Check sheet for the modelled part. Datum: model origin and axes. Units: mm. Give positions to 0.01 mm unless a question says otherwise; leave off trailing zeros. Order: outer loops, then holes, each group sorted by start corner. A loop starts at its lowest first (then second) coordinate and runs counter-clockwise, first axis right, second up.
from build123d import *

# Parameters (mm, degrees)
BOSS_EXTRUDE1_DEPTH = 4
CUT_EXTRUDE1_DEPTH  = 5


with BuildPart() as part:
    # Sketch1 → Boss-Extrude1 (new body)
    with BuildSketch(Plane(origin=(0, 0, 0), x_dir=(1, 0, 0), z_dir=(0, 1, 0))):
        Polygon((-65.5, 20), (-70, 20), (-70, -19.415515436), (-65.5, -19.415515436), (-65.5, -60), (65.5, -60), (65.5, -19.415515436), (70, -19.415515436), (70, 20), (65.5, 20), (65.5, 60), (-65.5, 60), align=None)
    extrude(amount=BOSS_EXTRUDE1_DEPTH)

    # Sketch2 → Cut-Extrude1 (cut)
    with BuildSketch(Plane(origin=(0, 4, 0), x_dir=(1, 0, 0), z_dir=(0, 1, 0))):
        with BuildLine():
            Line((-53.5, -20), (12.5, -20))
            ThreePointArc((12.5, -20), (13.914213562, -19.414213562), (14.5, -18))
            Line((14.5, -18), (14.5, 48))
            ThreePointArc((14.5, 48), (13.914213562, 49.414213562), (12.5, 50))
            Line((12.5, 50), (-53.5, 50))
            ThreePointArc((-53.5, 50), (-54.914213562, 49.414213562), (-55.5, 48))
            Line((-55.5, 48), (-55.5, -18))
            ThreePointArc((-55.5, -18), (-54.914213562, -19.414213562), (-53.5, -20))
        make_face()
        with BuildLine():
            Line((22.5, -44), (38.5, -44))
            ThreePointArc((38.5, -44), (39.207106781, -43.707106781), (39.5, -43))
            Line((39.5, -43), (39.5, -37))
            ThreePointArc((39.5, -37), (39.207106781, -36.292893219), (38.5, -36))
            Line((38.5, -36), (22.5, -36))
            ThreePointArc((22.5, -36), (21.792893219, -36.292893219), (21.5, -37))
            Line((21.5, -37), (21.5, -43))
            ThreePointArc((21.5, -43), (21.792893219, -43.707106781), (22.5, -44))
        make_face()
    extrude(amount=-CUT_EXTRUDE1_DEPTH, mode=Mode.SUBTRACT)


solid = part.part
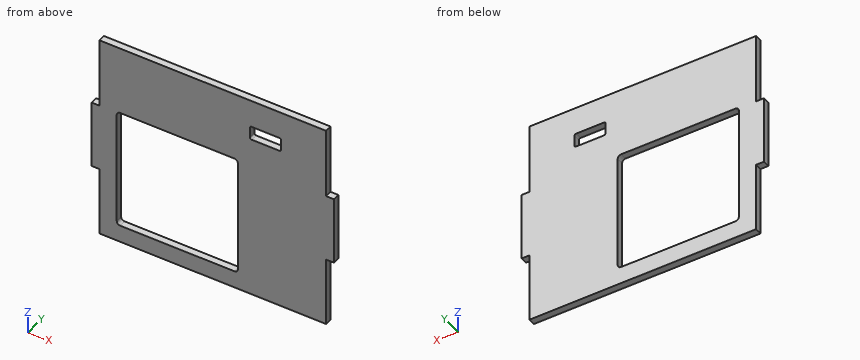
1) Depth check by flat-ended pin: pin 1 Ø1.2 at (y, z) = (3, -36) entering from +X; pin 2 Ø2 at (x, y) = (67, 1.5) entering from +Z; pin 3 Ø2 at (y, z) = (2, 48.5) entering from -X; pin 4 Ø8 at (x, z) = (8, -12) entering from +Y. Enter the tip coordinate at first touch or a pass-through.
Recorded:
pin 1: stops at x = 65.5
pin 2: stops at z = 19.42
pin 3: stops at x = -65.5
pin 4: passes through
2) Section check D-D, the plane z = 30. Record the cut outline in (x, y), then the cut area to 3 significant figures.
Recorded:
outline: (-65.5, 0) - (65.5, 0) - (65.5, 4) - (-65.5, 4) - close
area: 524 mm2
3) Section check C-C, the plane y = 2.1. Record the cut outline in (x, z).
Recorded:
outline: (-70, -20) - (-65.5, -20) - (-65.5, -60) - (65.5, -60) - (65.5, -20) - (70, -20) - (70, 19.42) - (65.5, 19.42) - (65.5, 60) - (-65.5, 60) - (-65.5, 19.42) - (-70, 19.42) - close; hole (-55.5, -48) arc R2 ccw to (-53.5, -50) - (12.5, -50) arc R2 ccw to (14.5, -48) - (14.5, 18) arc R2 ccw to (12.5, 20) - (-53.5, 20) arc R2 ccw to (-55.5, 18) - close; hole (21.5, 37) arc R1 ccw to (22.5, 36) - (38.5, 36) arc R1 ccw to (39.5, 37) - (39.5, 43) arc R1 ccw to (38.5, 44) - (22.5, 44) arc R1 ccw to (21.5, 43) - close
4) Material ranges on L1, parallel to X at y = 2.1, z = 12.5; L2, parallel to X at y = 2, z = -21; L3, parallel to Z at x = -27, y = 3.5, recorded low to high.
Recorded:
L1: x = -70 to -55.5, 14.5 to 70
L2: x = -65.5 to -55.5, 14.5 to 65.5
L3: z = -60 to -50, 20 to 60
5) Section check A-A, the plane x = -3.5. Record the cut outline in (y, z).
Recorded:
outline: (0, -60) - (4, -60) - (4, -50) - (0, -50) - close; (0, 20) - (4, 20) - (4, 60) - (0, 60) - close
6) Section check B-B, the plane z = -30. Record the cut outline in (x, y), then the cut area to 3 significant figures.
Recorded:
outline: (-65.5, 0) - (-55.5, 0) - (-55.5, 4) - (-65.5, 4) - close; (14.5, 0) - (65.5, 0) - (65.5, 4) - (14.5, 4) - close
area: 244 mm2
